Part model, mm, in its own coordinate system. Coordinates: 2 decimals unless noted, no trailing zeros. Write each loop counter-clockwise with the first axis right and the second up, starting at its lowest first coordinate (ties: lowest second). Pieces come first, ordered by that corner, then holes. Notation, with made-up numbers: (-14.5, 68) -> (22.5, 68) arc R22 ccw to (22.5, 75) -> close; hole circle Ø6 at (17.5, 20.5). An arc over 180 degrees is marked (long way). Write item = value, one per line. Start each with the question number.
Q1. Band-saw the part on A-A, the plane x = -14.5. List the corners of the cut face in (y, z) (3 decimals), plus the area to 3 significant figures.
Q2. Band-saw the part on C-C, the plane y = 1.1. Give the number of separate pieces and of enclosed holes in the cut face, plus the area to 3 significant figures.
Q3. Band-saw the part on B-B, the plane z = -27.5. List the corners of the cut face in (x, y) (3 decimals).
Q4. Probe line 1 (Z direction, x = -21.5, y = 0.85); line 2 (X direction, y = 1.2, z = -29.5); line 3 (Z direction, x = -19, y = 0.2) (3 decimals). List the from-to ranges inside material, lowest first.
Autodesk Inventor part; units mm, degrees
ref_plane "YZ Plane" through (0, 0, 0) normal (1, 0, 0) x (0, 1, 0)
ref_plane "XZ Plane" through (0, 0, 0) normal (0, 1, 0) x (-1, 0, 0)
ref_plane "XY Plane" through (0, 0, 0) normal (0, 0, 1) x (1, 0, 0)
sketch "Sketch1" plane through (0, 0, 0) normal (0, 1, 0) x (-1, 0, 0)
  line L0 (0, 0) -> (25, 0)
  line L1 (25, 0) -> (25, -76)
  line L2 (25, -76) -> (0, -76)
  line L3 (0, -76) -> (0, 0)
  dimension "d0" = 76
  dimension "d1" = 25
extrude "Extrusion1" add sketch "Sketch1" along normal blind 1.5
ref_plane "Work Plane2" through (0, 5.5, 0) normal (0, 1, 0) x (1, 0, 0)
sketch "Sketch3" plane through (0, 5.5, 0) normal (0, 1, 0) x (1, 0, 0)
  line L0 (0, 0) -> (-25, 0) construction
  line L1 (-12.5, 0) -> (-12.5, 76) construction
  line L2 (-25, 76) -> (0, 76) construction
  line L3 (-25, 71) -> (-25, 5) construction
  line L4 (-25, 38) -> (-0.4405, 38) construction
  line L5 (-20, 28.5) -> (-5, 28.5) construction
  line L6 (-3, 30.5) -> (-3, 45.5) construction
  line L7 (-5, 47.5) -> (-20, 47.5) construction
  line L8 (-22, 45.5) -> (-22, 30.5) construction
  line L9 (-22, 28.5) -> (-3, 47.5) construction
  line L10 (-3, 28.5) -> (-22, 47.5) construction
  arc A0 (-20, 47.5) -> (-22, 45.5) centre (-20, 45.5) ccw construction
  arc A1 (-3, 45.5) -> (-5, 47.5) centre (-5, 45.5) ccw construction
  arc A2 (-5, 28.5) -> (-3, 30.5) centre (-5, 30.5) ccw construction
  arc A3 (-22, 30.5) -> (-20, 28.5) centre (-20, 30.5) ccw construction
  line L11 (-22, 47.5) -> (-18, 47.5)
  line L12 (-18, 47.5) -> (-18, 43.5)
  line L13 (-18, 43.5) -> (-22, 43.5)
  line L14 (-22, 43.5) -> (-22, 47.5)
  line L15 (0, 47.5) -> (-15, 47.5) construction
  line L16 (-13, 43.5) -> (-17, 43.5)
  line L17 (-13, 47.5) -> (-13, 43.5)
  line L18 (-17, 47.5) -> (-13, 47.5)
  line L19 (-17, 43.5) -> (-17, 47.5)
  line L20 (5, 47.5) -> (-10, 47.5) construction
  line L21 (-8, 43.5) -> (-12, 43.5)
  line L22 (-8, 47.5) -> (-8, 43.5)
  line L23 (-12, 47.5) -> (-8, 47.5)
  line L24 (-12, 43.5) -> (-12, 47.5)
  line L25 (10, 47.5) -> (-5, 47.5) construction
  line L26 (-3, 43.5) -> (-7, 43.5)
  line L27 (-3, 47.5) -> (-3, 43.5)
  line L28 (-7, 47.5) -> (-3, 47.5)
  line L29 (-7, 43.5) -> (-7, 47.5)
  line L30 (-5, 42.5) -> (-20, 42.5) construction
  line L31 (-18, 38.5) -> (-22, 38.5)
  line L32 (-18, 42.5) -> (-18, 38.5)
  line L33 (-22, 42.5) -> (-18, 42.5)
  line L34 (-22, 38.5) -> (-22, 42.5)
  line L35 (0, 42.5) -> (-15, 42.5) construction
  line L36 (-13, 38.5) -> (-17, 38.5)
  line L37 (-13, 42.5) -> (-13, 38.5)
  line L38 (-17, 42.5) -> (-13, 42.5)
  line L39 (-17, 38.5) -> (-17, 42.5)
  line L40 (5, 42.5) -> (-10, 42.5) construction
  line L41 (-8, 38.5) -> (-12, 38.5)
  line L42 (-8, 42.5) -> (-8, 38.5)
  line L43 (-12, 42.5) -> (-8, 42.5)
  line L44 (-12, 38.5) -> (-12, 42.5)
  line L45 (10, 42.5) -> (-5, 42.5) construction
  line L46 (-3, 38.5) -> (-7, 38.5)
  line L47 (-3, 42.5) -> (-3, 38.5)
  line L48 (-7, 42.5) -> (-3, 42.5)
  line L49 (-7, 38.5) -> (-7, 42.5)
  line L50 (-5, 37.5) -> (-20, 37.5) construction
  line L51 (-18, 33.5) -> (-22, 33.5)
  line L52 (-18, 37.5) -> (-18, 33.5)
  line L53 (-22, 37.5) -> (-18, 37.5)
  line L54 (-22, 33.5) -> (-22, 37.5)
  line L55 (0, 37.5) -> (-15, 37.5) construction
  line L56 (-13, 33.5) -> (-17, 33.5)
  line L57 (-13, 37.5) -> (-13, 33.5)
  line L58 (-17, 37.5) -> (-13, 37.5)
  line L59 (-17, 33.5) -> (-17, 37.5)
  line L60 (5, 37.5) -> (-10, 37.5) construction
  line L61 (-8, 33.5) -> (-12, 33.5)
  line L62 (-8, 37.5) -> (-8, 33.5)
  line L63 (-12, 37.5) -> (-8, 37.5)
  line L64 (-12, 33.5) -> (-12, 37.5)
  line L65 (10, 37.5) -> (-5, 37.5) construction
  line L66 (-3, 33.5) -> (-7, 33.5)
  line L67 (-3, 37.5) -> (-3, 33.5)
  line L68 (-7, 37.5) -> (-3, 37.5)
  line L69 (-7, 33.5) -> (-7, 37.5)
  line L70 (-5, 32.5) -> (-20, 32.5) construction
  line L71 (-18, 28.5) -> (-22, 28.5)
  line L72 (-18, 32.5) -> (-18, 28.5)
  line L73 (-22, 32.5) -> (-18, 32.5)
  line L74 (-22, 28.5) -> (-22, 32.5)
  line L75 (0, 32.5) -> (-15, 32.5) construction
  line L76 (-13, 28.5) -> (-17, 28.5)
  line L77 (-13, 32.5) -> (-13, 28.5)
  line L78 (-17, 32.5) -> (-13, 32.5)
  line L79 (-17, 28.5) -> (-17, 32.5)
  line L80 (5, 32.5) -> (-10, 32.5) construction
  line L81 (-8, 28.5) -> (-12, 28.5)
  line L82 (-8, 32.5) -> (-8, 28.5)
  line L83 (-12, 32.5) -> (-8, 32.5)
  line L84 (-12, 28.5) -> (-12, 32.5)
  line L85 (10, 32.5) -> (-5, 32.5) construction
  line L86 (-3, 28.5) -> (-7, 28.5)
  line L87 (-3, 32.5) -> (-3, 28.5)
  line L88 (-7, 32.5) -> (-3, 32.5)
  line L89 (-7, 28.5) -> (-7, 32.5)
  point P0 (-12.5, 38)
  point P1 (2, 47.5)
  point P2 (7, 47.5)
  point P3 (12, 47.5)
  point P4 (-3, 42.5)
  point P5 (2, 42.5)
  point P6 (7, 42.5)
  point P7 (12, 42.5)
  point P8 (-3, 37.5)
  point P9 (2, 37.5)
  point P10 (7, 37.5)
  point P11 (12, 37.5)
  point P12 (-3, 32.5)
  point P13 (2, 32.5)
  point P14 (7, 32.5)
  point P15 (12, 32.5)
  dimension "d8" = 19
  dimension "d9" = 2
  dimension "d10" = 2
  dimension "d11" = 2
  dimension "d12" = 2
  dimension "d20" = 4
  dimension "d23" = 5
  dimension "d26" = 5
extrude "Extrusion3" cut sketch "Sketch3" against normal blind 6
sketch "Sketch4" plane through (0, 0, 0) normal (0, -1, 0) x (1, 0, 0)
  line L0 (0, -76) -> (0, 0) construction
  line L1 (0, -38) -> (-25, -38) construction
  line L2 (-25, -71) -> (-25, -5) construction
  line L3 (0, 0) -> (-25, 0) construction
  line L4 (-12.5, 0) -> (-12.5, -76) construction
  line L5 (-25, -76) -> (0, -76) construction
  line L6 (-19.875, -49.375) -> (-5.125, -49.375)
  line L7 (-1.125, -49.375) -> (-1.125, -26.625)
  line L8 (-5.125, -26.625) -> (-19.875, -26.625)
  line L9 (-23.875, -26.625) -> (-23.875, -49.375)
  line L10 (-23.875, -49.375) -> (-1.125, -26.625) construction
  line L11 (-1.125, -49.375) -> (-23.875, -26.625) construction
  arc A0 (-1.125, -26.625) -> (-5.125, -26.625) centre (-3.125, -26.625) ccw
  arc A1 (-19.875, -26.625) -> (-23.875, -26.625) centre (-21.875, -26.625) ccw
  arc A2 (-23.875, -49.375) -> (-19.875, -49.375) centre (-21.875, -49.375) ccw
  arc A3 (-5.125, -49.375) -> (-1.125, -49.375) centre (-3.125, -49.375) ccw
  point P0 (-12.5, -38)
  dimension "d15" = 22.75
  dimension "d16" = 4
  dimension "d17" = 22.75
extrude "Extrusion4" cut sketch "Sketch4" against normal blind 0.5
properties part number "scope coverslip holder lowpro offset"
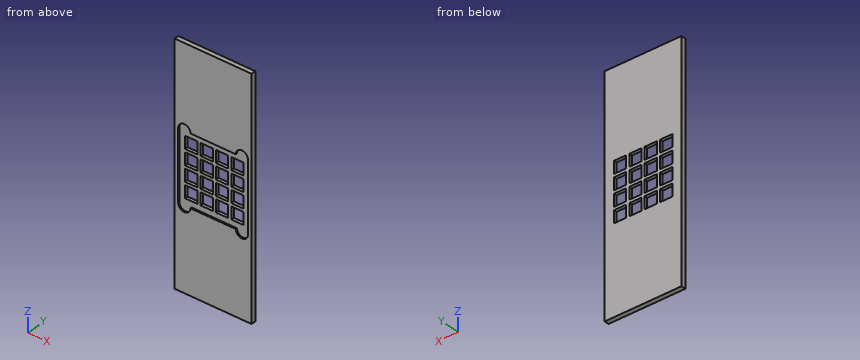
Ans:
q1.outline = (0, -76) -> (1.5, -76) -> (1.5, -47.5) -> (0.5, -47.5) -> (0.5, -49.375) -> (0, -49.375) -> close; (0, -26.625) -> (0.5, -26.625) -> (0.5, -28.5) -> (1.5, -28.5) -> (1.5, 0) -> (0, 0) -> close; (0.5, -43.5) -> (1.5, -43.5) -> (1.5, -42.5) -> (0.5, -42.5) -> close; (0.5, -38.5) -> (1.5, -38.5) -> (1.5, -37.5) -> (0.5, -37.5) -> close; (0.5, -33.5) -> (1.5, -33.5) -> (1.5, -32.5) -> (0.5, -32.5) -> close
q1.area = 86.6 mm2
q2.separate_pieces = 1
q2.enclosed_holes = 16
q2.area = 1,640 mm2
q3.outline = (-25, 0) -> (-23.875, 0) -> (-23.875, 0.5) -> (-1.125, 0.5) -> (-1.125, 0) -> (0, 0) -> (0, 1.5) -> (-25, 1.5) -> close
q4.line_1 = -76 to -47.5, -43.5 to -42.5, -38.5 to -37.5, -33.5 to -32.5, -28.5 to 0
q4.line_2 = -25 to -22, -18 to -17, -13 to -12, -8 to -7, -3 to 0
q4.line_3 = -76 to -49.375, -26.625 to 0
